```python
from build123d import *

# Parameters (mm, degrees)
SKETCH1_W           = 275
SKETCH1_H           = 90
BOSS_EXTRUDE1_DEPTH = 7
SKETCH2_R           = 4.05
CUT_EXTRUDE1_DEPTH  = 10


with BuildPart() as part:
    # Sketch1 → Boss-Extrude1 (new body)
    with BuildSketch(Plane.XY):
        with Locations((137.5, 45)):
            Rectangle(SKETCH1_W, SKETCH1_H)
    extrude(amount=BOSS_EXTRUDE1_DEPTH)

    # Sketch2 → Cut-Extrude1 (cut)
    with BuildSketch(Plane.XY.offset(7)):
        with Locations((265, 65)):
            Circle(SKETCH2_R)
        with Locations((265, 25)):
            Circle(SKETCH2_R)
        with Locations((215, 65)):
            Circle(SKETCH2_R)
        with Locations((215, 25)):
            Circle(SKETCH2_R)
        with Locations((165, 65)):
            Circle(SKETCH2_R)
        with Locations((165, 25)):
            Circle(SKETCH2_R)
        with Locations((115, 65)):
            Circle(SKETCH2_R)
        with Locations((115, 25)):
            Circle(SKETCH2_R)
        with Locations((65, 65)):
            Circle(SKETCH2_R)
        with Locations((65, 25)):
            Circle(SKETCH2_R)
        with Locations((265, 80)):
            Circle(SKETCH2_R)
        with Locations((265, 10)):
            Circle(SKETCH2_R)
        with Locations((215, 80)):
            Circle(SKETCH2_R)
        with Locations((215, 10)):
            Circle(SKETCH2_R)
        with Locations((165, 80)):
            Circle(SKETCH2_R)
        with Locations((165, 10)):
            Circle(SKETCH2_R)
        with Locations((115, 80)):
            Circle(SKETCH2_R)
        with Locations((115, 10)):
            Circle(SKETCH2_R)
        with Locations((65, 80)):
            Circle(SKETCH2_R)
        with Locations((65, 10)):
            Circle(SKETCH2_R)
        with Locations((15, 80)):
            Circle(SKETCH2_R)
        with Locations((15, 25)):
            Circle(SKETCH2_R)
        with Locations((15, 10)):
            Circle(SKETCH2_R)
        with Locations((15, 65)):
            Circle(SKETCH2_R)
    extrude(amount=-CUT_EXTRUDE1_DEPTH, mode=Mode.SUBTRACT)


solid = part.part
```
For this review, take the finished solid that the model builds, in its own axes (mm). Round coordinates to 2 decimals unless told otherwise and drop trailing zeros. Write each loop counter-clockwise with the first axis right and the second up, starting at its lowest first coordinate (ties: lowest second). Pieces come first, ordered by that corner, then holes. Notation, with made-up numbers: (10, 62.5) - (66, 62.5) arc R14 cw to (66, 70.5) - close; hole circle Ø1 at (57, -39.75). An arc over 180 degrees is marked (long way). Put each result on its own line as item: value.
Q1. Mouldability with a two-part tool opening along Y and no side actions: class faces 1 (the face through (136, 0, 3)), 2 (the face through (14.473, 69.016, 3.549)), 3 (the face through (275, 44, 3)) as released by +Y, released by -Y, zero draft, split by the parting line, or undercut.
Solved:
face 1: released by -Y
face 2: undercut
face 3: zero draft
Q2. We need section B-B (y = 80). Give the boundary of the cut face in (x, z), and give its area (3 significant figures).
Solved:
outline: (0, 0) - (10.95, 0) - (10.95, 7) - (0, 7) - close; (19.05, 0) - (60.95, 0) - (60.95, 7) - (19.05, 7) - close; (69.05, 0) - (110.95, 0) - (110.95, 7) - (69.05, 7) - close; (119.05, 0) - (160.95, 0) - (160.95, 7) - (119.05, 7) - close; (169.05, 0) - (210.95, 0) - (210.95, 7) - (169.05, 7) - close; (219.05, 0) - (260.95, 0) - (260.95, 7) - (219.05, 7) - close; (269.05, 0) - (275, 0) - (275, 7) - (269.05, 7) - close
area: 1,580 mm2
Q3. Insertion check: pin 1 Ø7.5 at (x, y) = (115, 25) entering from -Z. The pin has a flat end and moves straight along its axis. Give the tip position at first contact, or say it passes through.
Solved:
pin 1: passes through
Q4. We need section C-C (z = 4). Count the separate pieces of the cut face and the enclosed holes in it, and give its area (3 significant figures).
Solved:
separate pieces: 1
enclosed holes: 24
area: 23,500 mm2
Q5. Wall thickness on probe 1 along Y at (x, z) = (65, 5.5); probe 2 along Y at (x, z) = (67, 1.5): over which ranges is each line inside the solid? List them lowest first.
Solved:
probe 1: y = 0 to 5.95, 14.05 to 20.95, 29.05 to 60.95, 69.05 to 75.95, 84.05 to 90
probe 2: y = 0 to 6.48, 13.52 to 21.48, 28.52 to 61.48, 68.52 to 76.48, 83.52 to 90
Q6. We need section A-A (x = 165). Give the boundary of the cut face in (y, z), and give its area (3 significant figures).
Solved:
outline: (0, 0) - (5.95, 0) - (5.95, 7) - (0, 7) - close; (14.05, 0) - (20.95, 0) - (20.95, 7) - (14.05, 7) - close; (29.05, 0) - (60.95, 0) - (60.95, 7) - (29.05, 7) - close; (69.05, 0) - (75.95, 0) - (75.95, 7) - (69.05, 7) - close; (84.05, 0) - (90, 0) - (90, 7) - (84.05, 7) - close
area: 403 mm2
